Autodesk Inventor part; units mm, degrees
ref_plane "YZ Plane" through (0, 0, 0) normal (1, 0, 0) x (0, 1, 0)
ref_plane "XZ Plane" through (0, 0, 0) normal (0, 1, 0) x (-1, 0, 0)
sketch "Sketch1" plane through (0, 0, 0) normal (0, 1, 0) x (-1, 0, 0)
  circle A0 centre (0, 0) radius 14
  line L0 (0, 0) -> (9.779, 0) construction
  circle A1 centre (9.779, 0) radius 1.778
  circle A2 centre (6.9148, 6.9148) radius 1.778
  circle A3 centre (0, 9.779) radius 1.778
  circle A4 centre (-6.9148, 6.9148) radius 1.778
  circle A5 centre (-9.779, 0) radius 1.778
  circle A6 centre (-6.9148, -6.9148) radius 1.778
  circle A7 centre (0, -9.779) radius 1.778
  circle A8 centre (6.9148, -6.9148) radius 1.778
  dimension "d0" = 28
  dimension "d1" = 9.779
  dimension "d2" = 3.556
  dimension "d5" = 360
extrude "Extrusion1" add sketch "Sketch1" along normal blind 6.4
sketch "Sketch2" plane through (0, 6.4, 0) normal (0, 1, 0) x (1, 0, 0)
  circle A0 centre (0, 0) radius 6.25
  circle A1 centre (0, 0) radius 3
  dimension "d9" = 12.5
  dimension "d10" = 6
extrude "Extrusion2" add sketch "Sketch2" along normal blind 4
ref_plane "Work Plane1" through (0, 6.4, -6.25) normal (0, 0, 1) x (1, 0, 0)
sketch "Sketch3" plane through (0, 6.4, -6.25) normal (0, 0, 1) x (1, 0, 0)
  line L0 (-3, 4) -> (3, 4) construction
  line L1 (0, 4) -> (0, 0) construction
  line L2 (-1.778, 0) -> (1.778, 0) construction
  circle A0 centre (0, 2) radius 1.375
  point P0 (0, -6.4)
  dimension "d13" = 2.75
extrude "Extrusion3" cut sketch "Sketch3" along normal blind 1
sketch "Sketch4" plane through (0, 6.4, 0) normal (0, 1, 0) x (1, 0, 0)
  circle A0 centre (0, 0) radius 3
extrude "Extrusion4" cut sketch "Sketch4" against normal through all
properties part number "Main Motor to Sprocket Adapter"
The model under review builds one solid part; all positions refer to its coordinate system, in mm. A direction names the side the tool comes from. Round coordinates to 2 decimals unless told otherwise and drop trailing zeros. Write each loop counter-clockwise with the first axis right and the second up, starting at its lowest first coordinate (ties: lowest second). Pieces come first, ordered by that corner, then holes. Notation, with made-up numbers: M 41.5,71.25 L 50.5,71.25 A26 ccw 50.5,87.25 Z; hole C -33,-6.5 d9. An arc over 180 degrees is marked long. Answer as CSV lines item,"result". Start each with the question number.
Q1. Consider section A-A, the plane z = 0. Give the boundary of the cut face in (x, y).
Q2. Clearance check with flat-ended pins moving along their axes: P1, Ø3, axis at x = -6.5, y = 5.5, coming from the +Z side; P2, Ø1, axis at y = 7.5, z = 8.5, coming from the +X side; P3, Ø1.5, axis at x = -1.5, y = 2, coming from the +Z side; P4, Ø5.5, axis at x = -6.91, z = -6.91, coming from the +Y side. State where each tip first meets the part, or that it passes through.
Q3. Consider section D-D, the plane x = 3.75. Give the boundary of the cut face in (y, z).
Q4. Wall thickness on line 1 along Y through (x, z) = (0, -5.6) (3 decimals); line 2 along Z through (x, y) = (6, 5.5); line 3 along Y through (x, z) = (6.5, 1.75): over which ranges is each line inside the solid? List them lowest first.
Q5. Tool access review of faces 4 (the face through (0.2, 0, 3.3)), 5 (the face through (1.312, 7.987, -5.757)), 6 (the face through (-3, 6.4, -6)): name each direction out of +Z, -Z, +X, -X, +Y, -Y from which nothing blocks a thin tool from reaching the whole face with its end or side.
Q6. The part is to be moulded in two halves that separate along X. For faces 1 (the face through (-11.42, 3.16, 0.68)), 2 (the face through (-1, 10.4, 3)), 3 (the face through (3.36, 8.37, 5.27)), say which applies: +X half, -X half, draft (parallel to the pull), parting line (faces both ways), or undercut.
Q7. Consider section B-B, the plane x = 0. Give the boundary of the cut face in (y, z) (3 decimals).
Q8. Consider section C-C, the plane y = 8.4. Give the boundary of the cut face in (x, z) (3 decimals).
Result set:
1,outline,"M -14,0 L -11.56,0 L -11.56,6.4 L -14,6.4 Z; M -8,0 L -3,0 L -3,10.4 L -6.25,10.4 L -6.25,6.4 L -8,6.4 Z; M 3,0 L 8,0 L 8,6.4 L 6.25,6.4 L 6.25,10.4 L 3,10.4 Z; M 11.56,0 L 14,0 L 14,6.4 L 11.56,6.4 Z"
2,P1,"stops at z = 13.08"
2,P2,"passes through"
2,P3,"stops at z = 13.98"
2,P4,"stops at y = 6.4"
3,outline,"M 0,-13.49 L 6.4,-13.49 L 6.4,-5 L 10.4,-5 L 10.4,5 L 6.4,5 L 6.4,13.49 L 0,13.49 Z"
4,line 1,"y = 0 to 7.025, 9.775 to 10.4"
4,line 2,"z = -12.65 to -8.44, -5.39 to 5.39, 8.44 to 12.65"
4,line 3,"y = 0 to 6.4"
5,face 4,"+Z, -Z, +X, -X, -Y"
5,face 5,"-Z"
5,face 6,"+Y"
6,face 1,"undercut"
6,face 2,"draft"
6,face 3,"parting line"
7,outline,"M 0,-14 L 6.4,-14 L 6.4,-11.557 L 0,-11.557 Z; M 0,-8.001 L 6.4,-8.001 L 6.4,-6.25 L 7.025,-6.25 L 7.025,-5.25 L 9.775,-5.25 L 9.775,-6.25 L 10.4,-6.25 L 10.4,-3 L 0,-3 Z; M 0,3 L 10.4,3 L 10.4,6.25 L 6.4,6.25 L 6.4,8.001 L 0,8.001 Z; M 0,11.557 L 6.4,11.557 L 6.4,14 L 0,14 Z"
8,outline,"M -1.375,-6.097 L -1.375,-5.25 L 1.375,-5.25 L 1.375,-6.097 A6.25 ccw long Z; hole C 0,0 d6"
